```python
from build123d import *

# Parameters (mm, degrees)
F0_W     = 80
F0_H     = 40
F2_DEPTH = 3
F1_R     = 3
F1_W     = 12.9
F1_H     = 19.2
F3_DEPTH = 3.001
F4_R     = 1
F5_R     = 1.5
F6_DEPTH = 25


with BuildPart() as f2:
    # F0 (on Front) → F2 (new body)
    with BuildSketch(Plane.XZ):
        Rectangle(F0_W, F0_H)
    extrude(amount=F2_DEPTH)

    # F1 (on face) → F3 (cut, through all)
    with BuildSketch(Plane.XZ):
        with Locations((-28.43621, 10)):
            Circle(F1_R)
        with Locations((-28.43621, 0)):
            Circle(F1_R)
        with Locations((-28.43621, -10)):
            Circle(F1_R)
        with Locations((-18.43621, 10)):
            Circle(F1_R)
        with Locations((-18.43621, 0)):
            Circle(F1_R)
        with Locations((-18.43621, -10)):
            Circle(F1_R)
        with Locations((-8.43621, 10)):
            Circle(F1_R)
        with Locations((-8.43621, 0)):
            Circle(F1_R)
        with Locations((-8.43621, -10)):
            Circle(F1_R)
        with Locations((1.56379, 10)):
            Circle(F1_R)
        with Locations((1.56379, 0)):
            Circle(F1_R)
        with Locations((1.56379, -10)):
            Circle(F1_R)
        with Locations((11.56379, 10)):
            Circle(F1_R)
        with Locations((11.56379, 0)):
            Circle(F1_R)
        with Locations((11.56379, -10)):
            Circle(F1_R)
        with Locations((28.4711, -0.004033)):
            Rectangle(F1_W, F1_H)
    extrude(amount=F3_DEPTH, mode=Mode.SUBTRACT)

    # F4
    f4_edges = [f2.edges().sort_by_distance(p)[0] for p in [
        (-40, -1.5, 20),
        (40, -1.5, 20),
        (40, -1.5, -20),
        (-40, -1.5, -20),
    ]]
    fillet(f4_edges, radius=F4_R)

    # F5 (on face) → F6 (cut)
    with BuildSketch(Plane.XZ.offset(3)):
        with Locations((34.25, 14.25)):
            Circle(F5_R)
        with Locations((-34.25, -14.25)):
            Circle(F5_R)
    extrude(amount=-F6_DEPTH, mode=Mode.SUBTRACT)


solid = f2.part
```
Source: CAD feature listing. Evaluate the final solid. Frame: model axes, mm. A direction names the side the tool comes from. Give positions to 0.01 mm unless a question says otherwise; leave off trailing zeros. Order: outer loops, then holes, each group sorted by start corner. A loop starts at its lowest first (then second) coordinate and runs counter-clockwise, first axis right, second up.
(1) Section query A-A (z = 0). Return the cut outline in (x, y).
(2) Material intervals for line 1 along X through (y, z) = (-1.2, 10); line 2 along X through (y, z) = (-2.3, -6); line 3 along Z through (x, y) = (-18, -1.95), sorted ascending.
(3) Access query for faces 1 (the face through (34.921, -1, 0)), 2 (the face through (-40, -1, 0)). Directions: +Z, -Z, +X, -X, +Y, -Y. A direction counts if a zero-diameter tool reaches every point of the face in a straight line with its end or side. Return the directions, or none.
(4) Pull-direction query (Z, two-part tool) for faces 3 (the face through (4.425, -1.479, 10.901)), 4 (the face through (-1, -1, -20)), 5 (the face through (40, -1, 0)); classes: +Z half, -Z half, draft (parallel to the pull), parting line (faces both ways), or undercut.
(5) Contact query for a flat-ended pin moving along its axis: P1, Ø3.5, axis at x = -28.44, z = 0, coming from the -Y side. Output: stop coordinate, or through.
(6) Section query B-B (x = -34.25). Return the cut outline in (y, z).
(7) Section query D-D (z = -14.25). Return the cut outline in (x, y), plus the area to 3 significant figures.
(8) Section query C-C (y = -0.7). State how many separate pieces and enclosed holes the cut face has, plus the area to 3 significant figures.
Outcome:
1. outline: (-40, -3) - (-31.44, -3) - (-31.44, 0) - (-40, 0) - close; (-25.44, -3) - (-21.44, -3) - (-21.44, 0) - (-25.44, 0) - close; (-15.44, -3) - (-11.44, -3) - (-11.44, 0) - (-15.44, 0) - close; (-5.44, -3) - (-1.44, -3) - (-1.44, 0) - (-5.44, 0) - close; (4.56, -3) - (8.56, -3) - (8.56, 0) - (4.56, 0) - close; (14.56, -3) - (22.02, -3) - (22.02, 0) - (14.56, 0) - close; (34.92, -3) - (40, -3) - (40, 0) - (34.92, 0) - close
2. line 1: x = -40 to -31.44, -25.44 to -21.44, -15.44 to -11.44, -5.44 to -1.44, 4.56 to 8.56, 14.56 to 40
2. line 2: x = -40 to 22.02, 34.92 to 40
2. line 3: z = -20 to -12.97, -7.03 to -2.97, 2.97 to 7.03, 12.97 to 20
3. face 1: +Y, -Y
3. face 2: +Z, -Z, -X, +Y, -Y
4. face 3: undercut
4. face 4: -Z half
4. face 5: draft
5. P1: passes through
6. outline: (-3, -20) - (0, -20) - (0, -15.75) - (-3, -15.75) - close; (-3, -12.75) - (0, -12.75) - (0, 20) - (-3, 20) - close
7. outline: (-40, -3) - (-35.75, -3) - (-35.75, 0) - (-40, 0) - close; (-32.75, -3) - (40, -3) - (40, 0) - (-32.75, 0) - close
7. area: 231 mm2
8. separate pieces: 1
8. enclosed holes: 18
8. area: 2,510 mm2
